For this review, take the finished solid that the model builds, in its own axes (mm). A direction names the side the tool comes from. Give positions to 0.01 mm unless a question says otherwise; leave off trailing zeros. Write each loop counter-clockwise with the first axis right and the second up, starting at its lowest first coordinate (ties: lowest second). Pieces come first, ordered by that corner, then holes. Notation, with made-up numbers: M -20.75,55 L 26.25,55 A21 ccw 26.25,81 Z; hole C -27,40 d10. An arc over 180 degrees is marked long. Use one line per item in the form item = value. Start each with the question number.
Q1. Mouldability with a two-part tool opening along Z and no side actions: class faces 5 (the conical face through (-11.86, -68.6, 5.15)), 6 (the flat face through (26.79, 21.69, -1.15)), 7 (the cylindrical face through (10.65, 19.08, -8.48)), 8 (the flat face through (0.7, -67.8, 6)) as released by +Z, released by -Z, zero draft, split by the parting line, or undercut.
Q2. Consider section A-A on z = -6. Write out the cut boundary in (x, y).
Q3. Clearance check with flat-ended pins moving along their axes: pin 1 Ø10 at (x, y) = (4.32, -67.85) entering from -Z; pin 2 Ø4 at (x, z) = (21.5, -3.5) entering from -Y; pin 3 Ø5 at (x, y) = (18.32, -79.85) entering from -Z; pin 4 Ø8.5 at (x, y) = (4.32, -32.85) entering from +Z. State where each tip first meets the part, or that it passes through.
Q4. Consider section D-D on y = 8. Write out the cut boundary in (x, z).
Q5. Consider section C-C on x = -17. Write out the cut boundary in (y, z), and give its area (3 significant figures).
Q6. Consider section B-B on x = 18. Write out the cut boundary in (y, z), and give its area (3 significant figures).
Q7. Tool access review of faces 1 (the cylindrical face through (3.608, -71.067, 7.972)), 2 (the cylindrical face through (5.516, -38.215, 2.958)), 3 (the flat face through (20, -47, 6)), 4 (the cylindrical face through (-16.62, -67.21, 5.21)): name each direction out of +Z, -Z, +X, -X, +Y, -Y from which nothing blocks a thin tool from reaching the whole face with its end or side.
Q8. For probe 1 along Y at (x, z) = (5.5, 2.25); probe 2 along Y at (x, z) = (15.5, 6.5); probe 3 along Y at (x, z) = (2, 7), list the stretches that pass through material, from the lowest coordinate up. Write a range as [from, to].
```python
from build123d import *

# Parameters (mm, degrees)
SKETCH1_W             = 50
SKETCH1_H             = 112
SKETCH1_R             = 3.3
SKETCH1_R_2           = 2
SKETCH1_R_3           = 2.25
BOSS_EXTRUDE1_DEPTH   = 10
SKETCH2_R             = 5.5
CUT_EXTRUDE1_DEPTH    = 6
SKETCH3_R             = 4
CUT_EXTRUDE2_DEPTH    = 4
SKETCH4_W             = 50
SKETCH4_H             = 10
BOSS_EXTRUDE2_DEPTH   = 12
M4_TAPPED_HOLE1_D     = 3.3
M4_TAPPED_HOLE1_DEPTH = 8
M4_TAPPED_HOLE1_TIP   = 0.991420021
M4_TAPPED_HOLE2_D     = 3.3
M4_TAPPED_HOLE2_DEPTH = 8
M4_TAPPED_HOLE2_TIP   = 0.991420021
CHAMFER1_SIZE         = 5
M6_TAPPED_HOLE1_D     = 5
M6_TAPPED_HOLE1_DEPTH = 15
M6_TAPPED_HOLE1_TIP   = 1.502151548


with BuildPart() as part:
    # Sketch1 → Boss-Extrude1 (new body)
    with BuildSketch(Plane.XY):
        with Locations((4.323308271, -31.845864662)):
            Rectangle(SKETCH1_W, SKETCH1_H)
        with Locations((4.323308271, -67.845864662)):
            Circle(SKETCH1_R, mode=Mode.SUBTRACT)
        with Locations((4.323308271, -44.845864662)):
            Circle(SKETCH1_R_2, mode=Mode.SUBTRACT)
        with Locations((4.323308271, -32.845864662)):
            Circle(SKETCH1_R, mode=Mode.SUBTRACT)
        with Locations((18.323308271, -79.845864662)):
            Circle(SKETCH1_R_3, mode=Mode.SUBTRACT)
        with Locations((-9.676691729, -79.845864662)):
            Circle(SKETCH1_R_3, mode=Mode.SUBTRACT)
        with Locations((-9.676691729, -44.845864662)):
            Circle(SKETCH1_R_3, mode=Mode.SUBTRACT)
        with Locations((18.323308271, -44.845864662)):
            Circle(SKETCH1_R_3, mode=Mode.SUBTRACT)
        with Locations((4.323308271, -79.845864662)):
            Circle(SKETCH1_R_2, mode=Mode.SUBTRACT)
    extrude(amount=BOSS_EXTRUDE1_DEPTH)

    # Sketch2 → Cut-Extrude1 (cut)
    with BuildSketch(Plane(origin=(0, 0, 0), x_dir=(-1, 0, 0), z_dir=(0, 0, -1))):
        with Locations((-4.323308271, -32.845864662)):
            Circle(SKETCH2_R)
        with Locations((-4.323308271, -67.845864662)):
            Circle(SKETCH2_R)
    extrude(amount=-CUT_EXTRUDE1_DEPTH, mode=Mode.SUBTRACT)

    # Sketch3 → Cut-Extrude2 (cut)
    with BuildSketch(Plane.XY.offset(10)):
        with Locations((-9.676691729, -44.845864662)):
            Circle(SKETCH3_R)
        with Locations((18.323308271, -44.845864662)):
            Circle(SKETCH3_R)
        with Locations((18.323308271, -79.845864662)):
            Circle(SKETCH3_R)
        with Locations((-9.676691729, -79.845864662)):
            Circle(SKETCH3_R)
    extrude(amount=-CUT_EXTRUDE2_DEPTH, mode=Mode.SUBTRACT)

    # Sketch4 → Boss-Extrude2 (add)
    with BuildSketch(Plane(origin=(0, 0, 0), x_dir=(-1, 0, 0), z_dir=(0, 0, -1))):
        with Locations((-4.323308271, 19.154135338)):
            Rectangle(SKETCH4_W, SKETCH4_H)
    extrude(amount=BOSS_EXTRUDE2_DEPTH)

    # M4 Tapped Hole1
    with Locations(Plane(origin=(29.323308271, 0, 0), x_dir=(0, 0, -1), z_dir=(1, 0, 0))):
        with Locations((-5, -68.845864662)):
            Hole(M4_TAPPED_HOLE1_D / 2, depth=M4_TAPPED_HOLE1_DEPTH)
            with Locations((0, 0, -(M4_TAPPED_HOLE1_DEPTH + M4_TAPPED_HOLE1_TIP / 2))):  # 118° drill point
                Cone(0, M4_TAPPED_HOLE1_D / 2, M4_TAPPED_HOLE1_TIP, mode=Mode.SUBTRACT)

    # M4 Tapped Hole2
    with Locations(Plane.ZY.offset(20.676691729)):
        with Locations((5, -68.845864662)):
            Hole(M4_TAPPED_HOLE2_D / 2, depth=M4_TAPPED_HOLE2_DEPTH)
            with Locations((0, 0, -(M4_TAPPED_HOLE2_DEPTH + M4_TAPPED_HOLE2_TIP / 2))):  # 118° drill point
                Cone(0, M4_TAPPED_HOLE2_D / 2, M4_TAPPED_HOLE2_TIP, mode=Mode.SUBTRACT)

    # Chamfer1
    chamfer1_edges = [part.edges().sort_by_distance(p)[0] for p in [
        (-20.676691729, 24.154135338, -1),
        (29.323308271, 24.154135338, -1),
    ]]
    chamfer(chamfer1_edges, length=CHAMFER1_SIZE)

    # M6 Tapped Hole1
    with Locations(Plane(origin=(0, 24.154135338, 0), x_dir=(1, 0, 0), z_dir=(0, 1, 0))):
        with Locations((10.323308271, 6), (-1.676691729, 6)):
            Hole(M6_TAPPED_HOLE1_D / 2, depth=M6_TAPPED_HOLE1_DEPTH)
            with Locations((0, 0, -(M6_TAPPED_HOLE1_DEPTH + M6_TAPPED_HOLE1_TIP / 2))):  # 118° drill point
                Cone(0, M6_TAPPED_HOLE1_D / 2, M6_TAPPED_HOLE1_TIP, mode=Mode.SUBTRACT)


solid = part.part
```
Working result:
q1.face_5 = undercut
q1.face_6 = zero draft
q1.face_7 = undercut
q1.face_8 = released by -Z
q2.outline = M -20.68,14.15 L -4.18,14.15 L -4.18,24.15 L -15.68,24.15 L -20.68,19.15 Z; M 0.82,14.15 L 7.82,14.15 L 7.82,24.15 L 0.82,24.15 Z; M 12.82,14.15 L 29.32,14.15 L 29.32,19.15 L 24.32,24.15 L 12.82,24.15 Z
q3.pin_1 = 6
q3.pin_2 = 14.15
q3.pin_3 = 0
q3.pin_4 = 10
q4.outline = M -20.68,0 L 29.32,0 L 29.32,10 L -20.68,10 Z
q5.outline = M -87.85,0 L 14.15,0 L 14.15,-12 L 22.83,-12 L 22.83,10 L -87.85,10 Z; hole C -68.85,5 d3.3
q5.area = 1,200 mm²
q6.outline = M -87.85,0 L -82.07,0 L -82.07,6 L -83.83,6 L -83.83,10 L -87.85,10 Z; M -77.62,0 L -47.07,0 L -47.07,6 L -48.83,6 L -48.83,10 L -75.86,10 L -75.86,6 L -77.62,6 Z; M -42.62,0 L 14.15,0 L 14.15,-12 L 24.15,-12 L 24.15,10 L -40.86,10 L -40.86,6 L -42.62,6 Z
q6.area = 1,120 mm²
q7.face_1 = +Z, -Z
q7.face_2 = -Z
q7.face_3 = +Z
q7.face_4 = -X
q8.probe_1 = [-87.85, -81.46], [-78.23, -73.22], [-62.47, -46.46], [-43.23, -38.22], [-27.47, 24.15]
q8.probe_2 = [-87.85, -82.68], [-77.01, -47.68], [-42.01, 24.15]
q8.probe_3 = [-87.85, -70.19], [-65.5, -35.19], [-30.5, 24.15]
